Source: CAD feature listing. Evaluate the final solid. Frame: model axes, mm. A direction names the side the tool comes from. Give positions to 0.01 mm unless a question says otherwise; leave off trailing zeros. Order: outer loops, then holes, each group sorted by start corner. A loop starts at its lowest first (then second) coordinate and runs counter-clockwise, first axis right, second up. Notation, with made-up numbers: (3.25, 8) - (8.25, 8) arc R8 cw to (8.25, 18) - close; hole circle Ø7 at (-30.75, -35.75). An arc over 180 degrees is marked (long way). Write each question's results on one line, items separated by ' | '. Start each with the question number.
Item 1: Section C-C on z = 1.35. Output: boundary loops of the cut face in (x, y), and give its area (3 significant figures).
Item 2: Mould query, pull axis Y, two halves, no side actions, for faces 3 (the flat face through (0, 0, 0)), 4 (the cylindrical face through (4.479, -2.591, 0.538)), 5 (the cylindrical face through (2.96, -1.08, 4.88)). Classes: released by +Y, released by -Y, zero draft, split by the parting line, or undercut.
Item 3: Set-up query: faces 1 (the cylindrical face through (1.479, -2.468, 1.936)), 2 (the cylindrical face through (4.479, 0.326, -3.485)). Return all of +Z, -Z, +X, -X, +Y, -Y with unobstructed straight access to the full face (end or side cutting, diameter ignored); none if empty.
Item 4: Section A-A on y = 0. Output: boundary loops of the cut face in (x, z).
Item 5: Section D-D on x = 1.8. Output: boundary loops of the cut face in (y, z).
Item 6: Section B-B on z = -2.25. Output: boundary loops of the cut face in (x, y).
Item 7: Contact query for flat-ended pins moving along their axis: pin 1 Ø0.8 at (y, z) = (-2.5, 2) entering from +X; pin 2 Ø1 at (y, z) = (0, -2.7) entering from +X; pin 3 Ø2 at (x, z) = (1, 3.5) entering from +Y. Output: stop coordinate, or through.
Item 8: Line query: line 1 along Z through (x, y) = (4.65, 0); line 2 along Y through (x, z) = (1.05, 1.35); line 3 along Y through (x, z) = (3.5, 2). Output: solid intervals per line, ascending.
Autodesk Inventor part; units mm, degrees
ref_plane "YZ Plane" through (0, 0, 0) normal (1, 0, 0) x (0, 1, 0)
ref_plane "XZ Plane" through (0, 0, 0) normal (0, 1, 0) x (-1, 0, 0)
ref_plane "XY Plane" through (0, 0, 0) normal (0, 0, 1) x (1, 0, 0)
sketch "Эскиз1" plane through (0, 0, 0) normal (1, 0, 0) x (0, 1, 0)
  circle A0 centre (0, 0) radius 5
  circle A1 centre (0, -2.7) radius 0.6
  circle A2 centre (0, 0) radius 2.7 construction
  circle A3 centre (-2.3383, 1.35) radius 0.6
  circle A4 centre (2.3383, 1.35) radius 0.6
  line L0 (0, 0) -> (5.4782, 3.1628) construction
  line L1 (0, 0) -> (-5.2011, 3.0029) construction
  line L2 (0, 0) -> (5.5612, 0) construction
  dimension "d1" = 10
  dimension "d3" = 1.2
  dimension "d24" = 5.4
  dimension "d25" = 1.2
  dimension "d26" = 1.2
  dimension "d53" = 120
  dimension "d54" = 30
extrude "Выдавливание1" add sketch "Эскиз1" along normal blind 6 contours A0 | A3 | A4
hole "Отверстие2" at (6, 0, -2.7) direction (-1, 0, 0) diameter 1.7 depth 3
extrude "Выдавливание2" cut sketch "Эскиз1" along normal blind 6 contours A3 | A4
sketch "Эскиз2" plane through (6, 0, 0) normal (1, 0, 0) x (0, 0, -1)
  point P0 (0, 0)
  point P1 (-1.3483, 2.334)
hole "Отверстие4" at (6, 2.334, 1.3483) direction (-1, 0, 0) diameter 1.7 depth 3
sketch "Эскиз3" plane through (6, 0, 0) normal (1, 0, 0) x (0, 0, -1)
  point P0 (0, 0)
  point P1 (-1.3485, -2.336)
hole "Отверстие5" at (6, -2.336, 1.3485) direction (-1, 0, 0) diameter 1.7 depth 3
equation "\"d1\" = inside"
equation "\"d3\" = 2 * pin_small_rad"
equation "\"d17\" = pin_big_dia"
properties part number "каркас" material "Пластмасса, непрозрачная, черная"
Evaluation:
1) outline: (0, -4.81) - (6, -4.81) - (6, -3.19) - (3, -3.19) - (3, -2.94) - (0, -2.94) - close; (0, -1.74) - (3, -1.74) - (3, -1.49) - (6, -1.49) - (6, 1.48) - (3, 1.48) - (3, 1.74) - (0, 1.74) - close; (0, 2.94) - (3, 2.94) - (3, 3.18) - (6, 3.18) - (6, 4.81) - (0, 4.81) - close | area: 40.4 mm^2
2) face 3: zero draft | face 4: undercut | face 5: split by the parting line
3) face 1: +X, -X | face 2: +X
4) outline: (0, -5) - (6, -5) - (6, -3.55) - (3, -3.55) - (3, -3.3) - (0, -3.3) - close; (0, -2.1) - (3, -2.1) - (3, -1.85) - (6, -1.85) - (6, 5) - (0, 5) - close
5) outline: circle Ø10 at (0, 0); hole circle Ø1.2 at (-2.34, 1.35); hole circle Ø1.2 at (0, -2.7); hole circle Ø1.2 at (2.34, 1.35)
6) outline: (0, -4.47) - (6, -4.47) - (6, -0.72) - (3, -0.72) - (3, -0.4) - (0, -0.4) - close; (0, 0.4) - (3, 0.4) - (3, 0.72) - (6, 0.72) - (6, 4.47) - (0, 4.47) - close
7) pin 1: stops at x = 6 | pin 2: passes through | pin 3: stops at y = 4.33
8) line 1: z = -5 to -3.55, -1.85 to 5 | line 2: y = -4.81 to -2.94, -1.74 to 1.74, 2.94 to 4.81 | line 3: y = -4.58 to -2.88, -1.79 to 1.79, 2.88 to 4.58
